from build123d import *

# Parameters (mm, degrees)
SKETCH_1_W          = 42
SKETCH_1_H          = 42
EXTRUDE_1_DEPTH     = 8
SKETCH_2_R          = 9.5
CUT_EXTRUDE_1_DEPTH = 9
SKETCH_3_R          = 10.5
CUT_EXTRUDE_2_DEPTH = 5
SKETCH_6_R          = 11.05
CUT_EXTRUDE_3_DEPTH = 2
FILLET_1_R          = 4
SKETCH_8_R          = 19.5
CUT_EXTRUDE_4_DEPTH = 1
SKETCH_9_R          = 1.55
CUT_EXTRUDE_5_DEPTH = 9
SKETCH_10_R         = 1.55
CUT_EXTRUDE_6_DEPTH = 9
SKETCH_11_R         = 1.55
SKETCH_11_R_2       = 1.05
EXTRUDE_3_DEPTH     = 2


with BuildPart() as part:
    # 草图1 → 凸台-拉伸1 (new body)
    with BuildSketch(Plane.XY):
        Rectangle(SKETCH_1_W, SKETCH_1_H)
    extrude(amount=EXTRUDE_1_DEPTH)

    # 草图2 → 切除-拉伸1 (cut, through all)
    with BuildSketch(Plane.XY.offset(8)):
        Circle(SKETCH_2_R)
    extrude(amount=-CUT_EXTRUDE_1_DEPTH, mode=Mode.SUBTRACT)

    # 草图3 → 切除-拉伸2 (cut)
    with BuildSketch(Plane.XY.offset(8)):
        Circle(SKETCH_3_R)
    extrude(amount=-CUT_EXTRUDE_2_DEPTH, mode=Mode.SUBTRACT)

    # 草图6 → 切除-拉伸3 (cut)
    with BuildSketch(Plane(origin=(0, 0, 0), x_dir=(-1, 0, 0), z_dir=(0, 0, -1))):
        Circle(SKETCH_6_R)
    extrude(amount=-CUT_EXTRUDE_3_DEPTH, mode=Mode.SUBTRACT)

    # 圆角1
    fillet_1_edges = [part.edges().sort_by_distance(p)[0] for p in [
        (21, -21, 4),
        (-21, -21, 4),
        (-21, 21, 4),
        (21, 21, 4),
    ]]
    fillet(fillet_1_edges, radius=FILLET_1_R)

    # 草图8 → 切除-拉伸4 (cut)
    with BuildSketch(Plane.XY.offset(8)):
        Circle(SKETCH_8_R)
    extrude(amount=-CUT_EXTRUDE_4_DEPTH, mode=Mode.SUBTRACT)

    # 草图9 → 切除-拉伸5 (cut, through all)
    with BuildSketch(Plane(origin=(0, 0, 0), x_dir=(-1, 0, 0), z_dir=(0, 0, -1))):
        with Locations((-15.5, 15.5)):
            Circle(SKETCH_9_R)
        with Locations((15.5, 15.5)):
            Circle(SKETCH_9_R)
        with Locations((15.5, -15.5)):
            Circle(SKETCH_9_R)
        with Locations((-15.5, -15.5)):
            Circle(SKETCH_9_R)
    extrude(amount=-CUT_EXTRUDE_5_DEPTH, mode=Mode.SUBTRACT)

    # 草图10 → 切除-拉伸6 (cut, through all)
    with BuildSketch(Plane(origin=(0, 0, 0), x_dir=(-1, 0, 0), z_dir=(0, 0, -1))):
        with Locations((-18, 12)):
            Circle(SKETCH_10_R)
        with Locations((18, 12)):
            Circle(SKETCH_10_R)
        with Locations((18, -12)):
            Circle(SKETCH_10_R)
        with Locations((-18, -12)):
            Circle(SKETCH_10_R)
    extrude(amount=-CUT_EXTRUDE_6_DEPTH, mode=Mode.SUBTRACT)

    # 草图11 → 凸台-拉伸3 (add)
    with BuildSketch(Plane.XY.offset(8)):
        with Locations((-18, 12)):
            Circle(SKETCH_11_R)
        with Locations((-18, 12)):
            Circle(SKETCH_11_R_2, mode=Mode.SUBTRACT)
        with Locations((18, 12)):
            Circle(SKETCH_11_R)
        with Locations((18, 12)):
            Circle(SKETCH_11_R_2, mode=Mode.SUBTRACT)
        with Locations((18, -12)):
            Circle(SKETCH_11_R)
        with Locations((18, -12)):
            Circle(SKETCH_11_R_2, mode=Mode.SUBTRACT)
        with Locations((-18, -12)):
            Circle(SKETCH_11_R)
        with Locations((-18, -12)):
            Circle(SKETCH_11_R_2, mode=Mode.SUBTRACT)
    extrude(amount=-EXTRUDE_3_DEPTH)


solid = part.part
Can you work these out from the model? Positions are in its coordinate system, mm. A direction names the side the tool comes from. Give positions to 0.01 mm unless a question says otherwise; leave off trailing zeros. Write each loop counter-clockwise with the first axis right and the second up, starting at its lowest first coordinate (ties: lowest second). Pieces come first, ordered by that corner, then holes. Notation, with made-up numbers: (47.25, 81.5) -> (59.25, 81.5) arc R11 ccw to (59.25, 101.5) -> close; hole circle Ø3 at (-39.5, -18.75). An arc over 180 degrees is marked (long way). Answer as a JSON object with one key per item and string values. Group by question number.
Item 1: I'm going to push flat-ended pins straight in: P1, Ø6.5, axis at x = -5, y = -4.5, coming from the +Z side; P2, Ø1.9, axis at x = 18, y = 12, coming from the +Z side; P3, Ø4, axis at x = 15.5, y = -15.5, coming from the -Z side; P4, Ø1.6, axis at x = 18.5, y = -11.5, coming from the -Z side. Where does each tip first touch, or does it pass through?
Item 2: Please list where these lines run through material, in increasing order: line 1 (Y direction, x = 0, z = 4.9); line 2 (X direction, y = -12, z = 1.3); line 3 (Y direction, x = -18, z = 1.6). Write a range as [from, to].
Item 3: Suppose I cut it at D-D (y = -12.5). Please give me the cut outline in (x, z).
Item 4: We'd pull the mould along X, two halves only. Please class faces 1 (the face through (16.64, -14.45, 3.94)), 2 (the face through (-21, 0, 4)), 3 (the face through (0, 21, 4)), 4 (the face through (16.64, 16.55, 3.94)): +X half, -X half, draft (parallel to the pull), parting line (faces both ways), or undercut.
Item 5: Suppose I cut it at A-A (x = 0). Please give me the cut outline in (y, z).
Item 6: For faces 5 (the face through (-14.36, 16.55, 3.94)), 6 (the face through (10, 3.2, 5)), 7 (the face through (-19.432, -12.594, 2.958)), which set-ups out of +Z, -Z, +X, -X, +Y, -Y let a thin tool reach every point of the face, with its end or its side?
Item 7: Suppose I cut it at B-B (z = 7.5). State how many separate pieces and enclosed holes the cut face has, plus the area to 3 significant figures.
Findings:
{
 "1": {"P1": "stops at z = 3", "P2": "passes through", "P3": "stops at z = 0", "P4": "stops at z = 6"},
 "2": {"line 1": "y = [-21, -10.5], [10.5, 21]", "line 2": "x = [-21, -19.55], [-16.45, 16.45], [19.55, 21]", "line 3": "y = [-20.87, -13.55], [-10.45, 10.45], [13.55, 20.87]"},
 "3": {"outline": "(-21, 0) -> (-19.47, 0) -> (-19.47, 6) -> (-18.92, 6) -> (-18.92, 8) -> (-21, 8) -> close; (-17.08, 6) -> (-16.53, 6) -> (-16.53, 0) -> (16.53, 0) -> (16.53, 6) -> (17.08, 6) -> (17.08, 8) -> (14.97, 8) -> (14.97, 7) -> (-14.97, 7) -> (-14.97, 8) -> (-17.08, 8) -> close; (18.92, 6) -> (19.47, 6) -> (19.47, 0) -> (21, 0) -> (21, 8) -> (18.92, 8) -> close"},
 "4": {"face 1": "undercut", "face 2": "-X half", "face 3": "draft", "face 4": "undercut"},
 "5": {"outline": "(-21, 0) -> (-11.05, 0) -> (-11.05, 2) -> (-9.5, 2) -> (-9.5, 3) -> (-10.5, 3) -> (-10.5, 7) -> (-19.5, 7) -> (-19.5, 8) -> (-21, 8) -> close; (9.5, 2) -> (11.05, 2) -> (11.05, 0) -> (21, 0) -> (21, 8) -> (19.5, 8) -> (19.5, 7) -> (10.5, 7) -> (10.5, 3) -> (9.5, 3) -> close"},
 "6": {"face 5": "+Z, -Z", "face 6": "+Z", "face 7": "-Z"},
 "7": {"separate pieces": "1", "enclosed holes": "9", "area": "512 mm²"}
}
